Autodesk Inventor part; units mm, degrees
ref_plane "YZ Plane" through (0, 0, 0) normal (1, 0, 0) x (0, 1, 0)
ref_plane "XZ Plane" through (0, 0, 0) normal (0, 1, 0) x (-1, 0, 0)
ref_plane "XY Plane" through (0, 0, 0) normal (0, 0, 1) x (1, 0, 0)
sketch "Sketch1" plane through (0, 0, 0) normal (0, 0, 1) x (1, 0, 0)
  circle A0 centre (0, 0) radius 35.835
  circle A1 centre (0, 0) radius 29.715
  dimension "d0" = 71.67
  dimension "d1" = 59.43
extrude "Extrusion1" add sketch "Sketch1" along normal blind 180
thread "Thread1"
fillet "Fillet1" radius 1 2 edges at (-35.835, 0, 180) (-29.715, 0, 180)
fillet "Fillet2" radius 1 2 edges at (-29.715, 0, 0) (-35.835, 0, 0)
properties part number "4111_Bias_Coil_Layer2_MPSv2_v1" material "Copper"
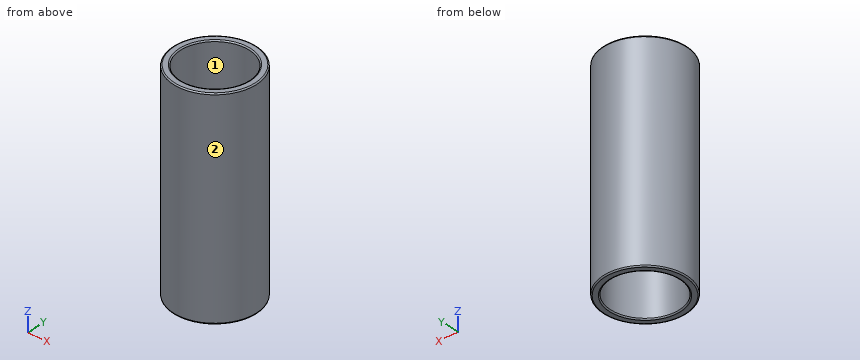
Geometry check sheet. Reference: the model listing, model coordinates, mm. Face numbers are marked on the shaded views. Give positions to 0.01 mm unless a question says otherwise; leave off trailing zeros. Order: outer loops, then holes, each group sorted by start corner. A loop starts at its lowest first (then second) coordinate and runs counter-clockwise, first axis right, second up.
1. Sectioned sample at C-C (z = 75.5). Record the boundary of the cut face in (x, y) (3 decimals).
Completed:
outline: circle Ø71.67 at (0, 0); hole circle Ø59.43 at (0, 0)
2. Depth check by flat-ended pin: pin 1 (1 mm diameter, centred on x = 1, z = 40, fed in from +Y); pin 2 (12 mm diameter, centred on y = -7.5, z = 63, fed in from +X); pin 3 (3 mm diameter, centred on x = -10.5, z = 96, fed in from -Y). Enter the tip coordinate at first touch or a pass-through.
Completed:
pin 1: stops at y = 35.83
pin 2: stops at x = 35.8
pin 3: stops at y = -34.69
3. Sectioned sample at A-A (x = 0). Record the boundary of the cut face in (y, z) (3 decimals).
Completed:
outline: (-35.835, 1) arc R1 ccw to (-34.835, 0) - (-30.715, 0) arc R1 ccw to (-29.715, 1) - (-29.715, 179) arc R1 ccw to (-30.715, 180) - (-34.835, 180) arc R1 ccw to (-35.835, 179) - close; (29.715, 1) arc R1 ccw to (30.715, 0) - (34.835, 0) arc R1 ccw to (35.835, 1) - (35.835, 179) arc R1 ccw to (34.835, 180) - (30.715, 180) arc R1 ccw to (29.715, 179) - close
4. Scan lines: line 1 (Y direction, x = 0, z = 115) (3 decimals); line 2 (X direction, y = 19.5, z = 82); line 3 (X direction, y = -17, z = 20.5). Record each from-to range of solid material in increasing order.
Completed:
line 1: y = -35.835 to -29.715, 29.715 to 35.835
line 2: x = -30.06 to -22.42, 22.42 to 30.06
line 3: x = -31.55 to -24.37, 24.37 to 31.55
5. Draft check along X on the marked faces 1 and 2. Enter one of: pulls with the +X half, pulls with the -X half, needs draft (parallel to the pull), parting line crosses it, or undercut.
Completed:
face 1: undercut
face 2: parting line crosses it
